Geometry check sheet. Reference: the model listing, model coordinates, mm. Coordinates: 2 decimals unless noted, no trailing zeros. Write each loop counter-clockwise with the first axis right and the second up, starting at its lowest first coordinate (ties: lowest second). Pieces come first, ordered by that corner, then holes. Notation, with made-up numbers: (-9.75, -10) -> (23.25, -10) arc R17 ccw to (23.25, 13) -> close; hole circle Ø8 at (-10, 25.5). An arc over 180 degrees is marked (long way). Answer in a Markdown table with one row per item. Add a question column.
1. Cross-section at D-D on y = 34.5. Record the cut outline in (x, z), and give its area (3 significant figures).
2. Scan lines: L1, parallel to Y at x = 2.5, z = 0; L2, parallel to Z at x = 1.2, y = -26; L3, parallel to Z at x = 1.8, y = -22.5. Record each from-to range of solid material in increasing order. Write a range as from..to.
3. Depth check by flat-ended pin: P1, Ø0.9, axis at x = 1.5, z = -36.5, coming from the -Y side; P2, Ø1.5, axis at x = 2, z = -36.5, coming from the +Y side; P3, Ø1, axis at x = 1, z = 24.5, coming from the -Y side. Enter the tip coordinate at first touch or a pass-through.
4. Cross-section at A-A on z = 0. Record the cut outline in (x, y), and give its area (3 significant figures).
5. Cross-section at B-B on y = 50. Record the cut outline in (x, z).
6. Cross-section at C-C on x = 0.6. Give the number of separate pieces and of enclosed holes in the cut face, and give its area (3 significant figures).
```python
from build123d import *

# Parameters (mm, degrees)
SKETCH1_R           = 57.5
BOSS_EXTRUDE1_DEPTH = 4
SKETCH2_R           = 4.25
CUT_EXTRUDE1_DEPTH  = 82.415600471
CUT_EXTRUDE2_DEPTH  = 82.415600471
CUT_EXTRUDE3_DEPTH  = 82.415600471


with BuildPart() as part:
    # Sketch1 → Boss-Extrude1 (new body)
    with BuildSketch(Plane(origin=(0, 0, 0), x_dir=(0, 0, -1), z_dir=(1, 0, 0))):
        Circle(SKETCH1_R)
    extrude(amount=BOSS_EXTRUDE1_DEPTH)

    # Sketch2 → Cut-Extrude1 (cut, through all)
    with BuildSketch(Plane.ZY):
        with Locations((0, 50)):
            Circle(SKETCH2_R)
        with Locations((43.301270189, -25)):
            Circle(SKETCH2_R)
        with Locations((-43.301270189, -25)):
            Circle(SKETCH2_R)
    extrude(amount=-CUT_EXTRUDE1_DEPTH, mode=Mode.SUBTRACT)

    # Sketch3 → Cut-Extrude2 (cut, through all)
    with BuildSketch(Plane.ZY):
        with BuildLine():
            Line((-30, -49.053542176), (-30, -24.053542176))
            Line((-30, -24.053542176), (30, -24.053542176))
            Line((30, -24.053542176), (30, -49.053542176))
            ThreePointArc((30, -49.053542176), (0, -57.5), (-30, -49.053542176))
        make_face()
    extrude(amount=-CUT_EXTRUDE2_DEPTH, mode=Mode.SUBTRACT)

    # Sketch4 → Cut-Extrude3 (cut, through all)
    with BuildSketch(Plane(origin=(4, 0, 0), x_dir=(0, 0, -1), z_dir=(1, 0, 0))):
        Polygon((15.999329975, 38.578303843), (18.05316756, 38.897288443), (18.803837585, 40.835456267), (17.500670025, 42.454639491), (15.44683244, 42.13565489), (14.696162415, 40.197487066), align=None)
        Polygon((-17.524724067, 38.587792684), (-15.467077039, 38.881201452), (-14.692352971, 40.809880435), (-15.975275933, 42.44515065), (-18.032922961, 42.151741882), (-18.807647029, 40.223062899), align=None)
        Polygon((15.975275933, 20.587792684), (18.032922961, 20.881201452), (18.807647029, 22.809880435), (17.524724067, 24.44515065), (15.467077039, 24.151741882), (14.692352971, 22.223062899), align=None)
        Polygon((-17.245318548, 20.646539693), (-15.172985813, 20.806029616), (-14.27494177, 22.680467371), (-15.449230462, 24.395415203), (-17.521563197, 24.235925281), (-18.41960724, 22.361487526), align=None)
        Polygon((33.9977786, 17.342133915), (35.4988893, 14.742133915), (38.5011107, 14.742133915), (40.0022214, 17.342133915), (38.5011107, 19.942133915), (35.4988893, 19.942133915), align=None)
        Polygon((-40.0022214, 17.342133915), (-38.5011107, 14.742133915), (-35.4988893, 14.742133915), (-33.9977786, 17.342133915), (-35.4988893, 19.942133915), (-38.5011107, 19.942133915), align=None)
        Polygon((-1.657389197, -17.116294048), (1.339206641, -17.299996833), (2.996595839, -14.796720104), (1.657389197, -12.109740591), (-1.339206641, -11.926037806), (-2.996595839, -14.429314535), align=None)
    extrude(amount=-CUT_EXTRUDE3_DEPTH, mode=Mode.SUBTRACT)


solid = part.part
```
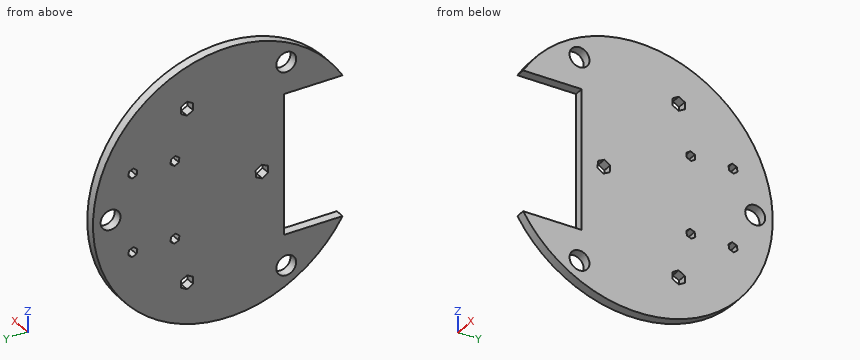
Results found:
| question | item | result |
|---|---|---|
| 1 | outline | (0, -46) -> (4, -46) -> (4, 46) -> (0, 46) -> close |
| 1 | area | 368 mm^2 |
| 2 | L1 | y = -24.05..-17.22, -12.01..45.75, 54.25..57.5 |
| 2 | L2 | z = -51.29..-47.43, -39.17..-30, 30..39.17, 47.43..51.29 |
| 2 | L3 | z = -52.92..-46.74, -39.86..39.86, 46.74..52.92 |
| 3 | P1 | stops at y = -44.8 |
| 3 | P2 | stops at y = 45.04 |
| 3 | P3 | stops at y = -24.05 |
| 4 | outline | (0, -24.05) -> (4, -24.05) -> (4, -17.22) -> (0, -17.22) -> close; (0, -12.01) -> (4, -12.01) -> (4, 45.75) -> (0, 45.75) -> close; (0, 54.25) -> (4, 54.25) -> (4, 57.5) -> (0, 57.5) -> close |
| 4 | area | 271 mm^2 |
| 5 | outline | (0, -28.39) -> (4, -28.39) -> (4, -4.25) -> (0, -4.25) -> close; (0, 4.25) -> (4, 4.25) -> (4, 28.39) -> (0, 28.39) -> close |
| 6 | separate pieces | 1 |
| 6 | enclosed holes | 10 |
| 6 | area | 8,260 mm^2 |
